Autodesk Inventor part; units mm, degrees
ref_plane "YZ Plane" through (0, 0, 0) normal (1, 0, 0) x (0, 1, 0)
ref_plane "XZ Plane" through (0, 0, 0) normal (0, 1, 0) x (-1, 0, 0)
ref_plane "XY Plane" through (0, 0, 0) normal (0, 0, 1) x (1, 0, 0)
ref_plane "작업 평면1" through (0, 0, -188.9899) normal (0, 0, 1) x (-0.9797373, 0.2002869, 0)
sketch "스케치1" plane through (0, 0, -188.9899) normal (0, 0, 1) x (-0.9797373, 0.2002869, 0)
  circle A0 centre (0, 0) radius 13.8
  circle A1 centre (0, 0) radius 7.2
  circle A2 centre (0, -11) radius 1.2813
  circle A3 centre (-7.7782, -7.7782) radius 1.2813
  circle A4 centre (-11, 0) radius 1.2813
  circle A5 centre (-7.7782, 7.7782) radius 1.2813
  circle A6 centre (0, 11) radius 1.2813
  circle A7 centre (7.7782, 7.7782) radius 1.2813
  circle A8 centre (11, 0) radius 1.2813
  circle A9 centre (7.7782, -7.7782) radius 1.2813
  line L0 (-17.5, -17.5) -> (17.5, -17.5)
  line L1 (17.5, -17.5) -> (17.5, 17.5)
  line L2 (17.5, 17.5) -> (-17.5, 17.5)
  line L3 (-17.5, 17.5) -> (-17.5, -17.5)
  line L4 (-17.5, -17.5) -> (17.5, 17.5) construction
  line L5 (17.5, -17.5) -> (-17.5, 17.5) construction
  circle A10 centre (0, 0) radius 7.3
  circle A11 centre (-11, 0) radius 1.3813
  circle A12 centre (-7.7782, 7.7782) radius 1.3813
  circle A13 centre (0, 11) radius 1.3813
  circle A14 centre (7.7782, 7.7782) radius 1.3813
  circle A15 centre (11, 0) radius 1.1813
  circle A16 centre (7.7782, -7.7782) radius 1.3813
  circle A17 centre (0, -11) radius 1.3813
  circle A18 centre (-7.7782, -7.7782) radius 1.3813
  line L6 (17.2724, -17.5) -> (17.2724, -18.1)
  line L7 (17.1076, 17.5) -> (17.1076, 22.85)
  line L8 (17.1076, 17.5) -> (22.4576, 17.5) construction
  line L9 (17.5, 22.85) -> (16.9, 22.85)
  line L10 (16.9, 22.85) -> (16.9, -18.1)
  line L11 (16.9, -18.1) -> (17.5, -18.1)
  line L12 (17.5, -18.1) -> (17.5, 22.85)
  line L13 (17.5, -18.1) -> (-17.5, -18.1)
  line L14 (-17.5, -18.1) -> (-17.5, 22.85)
  line L15 (-17.5, 22.85) -> (17.5, 22.85)
  line L16 (17.5, 22.85) -> (17.5, -18.1)
  line L17 (17.5, 17.5) -> (18.1, 17.5)
  line L18 (18.1, 17.5) -> (18.1, -17.5)
  line L19 (18.1, -17.5) -> (17.5, -17.5)
  line L20 (17.5, -17.5) -> (17.5, 17.5)
  line L21 (-17.5, 17.5) -> (-22.85, 17.5)
  line L22 (-22.85, 17.5) -> (-22.85, 15.9604)
  line L23 (-22.85, 15.9604) -> (-17.5, 15.9604)
  line L24 (-17.5, 15.9604) -> (-17.5, 17.5)
  line L25 (-22.85, 17.5) -> (-17.5, 17.5)
  line L26 (-17.5, 17.5) -> (-17.5, -17.5)
  line L27 (-17.5, -17.5) -> (-22.85, -17.5)
  line L28 (-22.85, -17.5) -> (-22.85, 17.5)
  point P0 (0, 0)
  point P1 (17.5, -17.5)
  point P2 (-17.5, -17.5)
  point P3 (16.9, -18.1)
  point P4 (16.9, 22.85)
  point P5 (-17.5, 17.5)
  point P6 (17.5, 17.5)
  point P7 (-22.85, 15.9604)
  point P8 (17.5, -17.5)
  dimension "d0" = 35
  dimension "d1" = 35
  dimension "d2" = 0.1
  dimension "d3" = 0.1
  dimension "d4" = 0.1
  dimension "d5" = 0.1
  dimension "d6" = 0.1
  dimension "d7" = 0.1
  dimension "d8" = 0.1
  dimension "d9" = 0.1
  dimension "d10" = 0.1
  dimension "d13" = 0.6
  dimension "d14" = 5.35
  dimension "d15" = 90
  dimension "d16" = 0.6
  dimension "d17" = 5.35
extrude "돌출1" add sketch "스케치1" along normal blind 6 contours A0 | L0 L10 L2 L1 | L1 L17 L18 L19 | L0 L3 L2 L10 | L27 L28 L23 L3 | L23 L22 L21 L3
sketch "스케치3" plane through (25.892, 12.5688, -182.9899) normal (0.9797373, -0.2002869, 0) x (0, 0, -1)
  circle A0 centre (2.59, -25.3) radius 1.55
  circle A1 centre (2.59, -9.7) radius 1.55
  line L0 (-34, -31.3) -> (6, -31.3)
  line L1 (6, -31.3) -> (6, -3.7)
  line L2 (6, -3.7) -> (-34, -3.7)
  arc A2 (-34, -3.7) -> (-34, -31.3) centre (-34, -17.5) ccw
  circle A3 centre (-41.7782, -25.2782) radius 1.65
  circle A4 centre (-45, -17.5) radius 1.65
  circle A5 centre (-41.7782, -9.7218) radius 1.65
  circle A6 centre (-34, -6.5) radius 1.65
  circle A7 centre (-26.2218, -9.7218) radius 1.65
  circle A8 centre (-23, -17.5) radius 1.65
  circle A9 centre (-26.2218, -25.2782) radius 1.65
  circle A10 centre (-34, -28.5) radius 1.65
  circle A11 centre (-34, -17.5) radius 5.1
  circle A12 centre (-34, -17.5) radius 3.9
  circle A13 centre (-34, -17.5) radius 4
  circle A14 centre (-28.3126, -11.8739) radius 1.2
  circle A15 centre (-39.6261, -11.8126) radius 1.2
  circle A16 centre (-39.6874, -23.1261) radius 1.2
  circle A17 centre (-28.3739, -23.1874) radius 1.2
  circle A18 centre (-34, -17.5) radius 4
  circle A19 centre (-34, -17.5) radius 10.9
  circle A20 centre (-34.0433, -25.4999) radius 1.2
  circle A21 centre (-41.9999, -17.4567) radius 1.2
  circle A22 centre (-33.9567, -9.5001) radius 1.2
  circle A23 centre (-26.0001, -17.5433) radius 1.2
  circle A24 centre (-34, -17.5) radius 3.5
  circle A25 centre (-34, -17.5) radius 5.2
  circle A26 centre (-26.0001, -17.5433) radius 1.3
  circle A27 centre (-28.3739, -23.1874) radius 1.3
  circle A28 centre (-34.0433, -25.4999) radius 1.3
  circle A29 centre (-39.6874, -23.1261) radius 1.3
  circle A30 centre (-41.9999, -17.4567) radius 1.3
  circle A31 centre (-39.6261, -11.8126) radius 1.3
  circle A32 centre (-33.9567, -9.5001) radius 1.3
  circle A33 centre (-28.3126, -11.8739) radius 1.3
  point P0 (-182.9899, -17.5)
  dimension "d22" = 0.1
  dimension "d23" = 0.1
  dimension "d24" = 0.1
  dimension "d25" = 0.1
  dimension "d26" = 0.1
  dimension "d27" = 0.1
  dimension "d28" = 0.1
  dimension "d29" = 0.1
  dimension "d30" = 0.1
  dimension "d31" = 0.1
extrude "돌출2" add sketch "스케치3" along normal blind 6 contours A0 | A1 | A2 L2 L1 L0 | A3 A19 | A3 A19 A4 A5 A6 A7 A8 A9 A10 | A19 A3 | A19 A4 | A4 A19 | A19 A10 | A10 A19 | A19 A5 | A5 A19 | A19 A9 | A9 A19 | A19 A6 | A6 A19 | A19 A8 | A8 A19 | A19 A7 | A7 A19 | A11 | A25
sketch "스케치4" plane through (-21.2383, -13.5202, -188.9899) normal (-0.9797373, 0.2002869, 0) x (0, 0, 1)
  circle A0 centre (3.41, 9.7) radius 1.55
  circle A1 centre (3.41, 25.3) radius 1.55
  line L0 (40, 3.7) -> (0, 3.7)
  arc A2 (40, 3.7) -> (40, 31.3) centre (40, 17.5) ccw
  line L1 (0, 31.3) -> (40, 31.3)
  line L2 (0, 3.7) -> (0, 31.3)
  circle A3 centre (47.7782, 9.7218) radius 1.65
  circle A4 centre (51, 17.5) radius 1.65
  circle A5 centre (47.7782, 25.2782) radius 1.65
  circle A6 centre (40, 28.5) radius 1.65
  circle A7 centre (32.2218, 25.2782) radius 1.65
  circle A8 centre (29, 17.5) radius 1.65
  circle A9 centre (32.2218, 9.7218) radius 1.65
  circle A10 centre (40, 6.5) radius 1.65
  circle A11 centre (40, 17.5) radius 5.1
  circle A12 centre (40, 17.5) radius 10.8
  circle A13 centre (40, 17.5) radius 6
  circle A14 centre (47.9984, 17.6612) radius 1.05
  circle A15 centre (45.7697, 11.9583) radius 1.05
  circle A16 centre (40.1612, 9.5016) radius 1.05
  circle A17 centre (34.4583, 11.7303) radius 1.05
  circle A18 centre (32.0016, 17.3388) radius 1.05
  circle A19 centre (34.2303, 23.0417) radius 1.05
  circle A20 centre (39.8388, 25.4984) radius 1.05
  circle A21 centre (45.5417, 23.2697) radius 1.05
  circle A22 centre (39.8388, 25.4984) radius 1.15
  circle A23 centre (34.2303, 23.0417) radius 1.15
  circle A24 centre (32.0016, 17.3388) radius 1.15
  circle A25 centre (34.4583, 11.7303) radius 1.15
  circle A26 centre (40.1612, 9.5016) radius 1.15
  circle A27 centre (45.7697, 11.9583) radius 1.15
  circle A28 centre (47.9984, 17.6612) radius 1.15
  circle A29 centre (45.5417, 23.2697) radius 1.15
  point P0 (188.9899, 17.5)
  dimension "d32" = 0.1
  dimension "d33" = 0.1
  dimension "d34" = 0.1
  dimension "d35" = 0.1
  dimension "d36" = 0.1
  dimension "d37" = 0.1
  dimension "d38" = 0.1
  dimension "d39" = 0.1
extrude "돌출3" add sketch "스케치4" along normal blind 6 contours A0 | A1 | L0 L2 L1 A2 | A3 A12 | A12 A3 | A3 A12 A10 A9 A8 A7 A6 A5 A4 | A12 A4 | A4 A12 | A12 A10 | A10 A12 | A12 A5 | A5 A12 | A12 A9 | A9 A12 | A12 A6 | A6 A12 | A12 A8 | A8 A12 | A12 A7 | A7 A12 | A13
sketch "스케치5" plane through (0, 0, -182.9899) normal (0, 0, 1) x (0.9797373, -0.2002869, 0)
  line L0 (22.85, 13.8) -> (22.85, -13.8)
  line L1 (22.85, -13.8) -> (28.85, -13.8)
  line L2 (28.85, 13.8) -> (28.85, -13.8)
  line L3 (22.85, 13.8) -> (28.85, 13.8)
  line L4 (-18.1, -13.8) -> (-18.1, 13.8)
  line L5 (-18.1, 13.8) -> (-24.1, 13.8)
  line L6 (-24.1, -13.8) -> (-24.1, 13.8)
  line L7 (-18.1, -13.8) -> (-24.1, -13.8)
  line L8 (22.85, -17.5) -> (22.85, -13.8)
  line L9 (-18.1, -13.8) -> (-18.1, -17.5)
  line L10 (22.85, -13.8) -> (-18.1, -13.8)
  line L11 (-18.1, -13.8) -> (-18.1, -17.5)
  line L12 (-18.1, -17.5) -> (22.85, -17.5)
  line L13 (22.85, -17.5) -> (22.85, -13.8)
  line L14 (-18.1, -17.5) -> (22.85, -17.5)
  line L15 (22.85, -17.5) -> (22.85, -13.8)
  line L16 (22.85, -13.8) -> (22.85, 13.8)
  line L17 (22.85, 13.8) -> (22.85, 17.5)
  line L18 (22.85, 17.5) -> (-18.1, 17.5)
  line L19 (-18.1, 17.5) -> (-18.1, 13.8)
  line L20 (-18.1, 13.8) -> (-18.1, -13.8)
  line L21 (-18.1, -13.8) -> (-18.1, -17.5)
  circle A0 centre (-11, 0) radius 1.2813
  circle A1 centre (0, 0) radius 7.3
  circle A2 centre (11, 0) radius 1.3813
  circle A3 centre (7.7782, -7.7782) radius 1.3813
  circle A4 centre (0, -11) radius 1.3813
  circle A5 centre (-7.7782, -7.7782) radius 1.3813
  circle A6 centre (-7.7782, 7.7782) radius 1.3813
  circle A7 centre (0, 11) radius 1.3813
  circle A8 centre (7.7782, 7.7782) radius 1.3813
  line L22 (22.85, 13.8) -> (-18.3673, 13.8)
  line L23 (-18.3673, 13.8) -> (-18.3673, 17.5)
  line L24 (-18.3673, 17.5) -> (22.85, 17.5)
  line L25 (22.85, 17.5) -> (22.85, 13.8)
  point P0 (0, 0)
  point P1 (-18.1, 13.8)
  point P2 (-18.1, -13.8)
  point P3 (22.85, -17.5)
extrude "돌출4" cut sketch "스케치5" against normal blind 10 contours L22 L19 L18 L17 | L8 L12 L9 L10
properties part number "37" material "LCP 플라스틱"
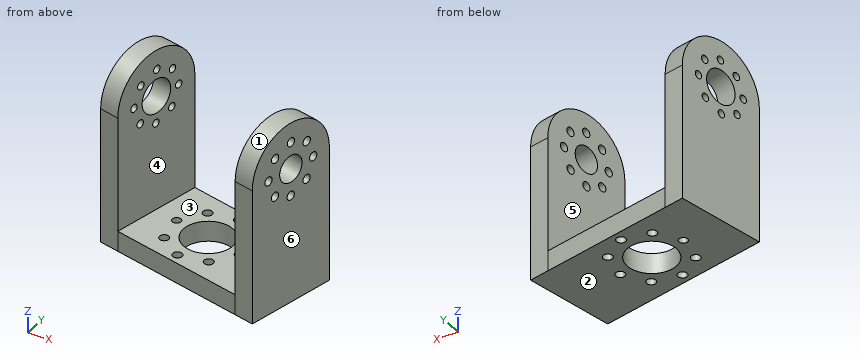
Source: CAD feature listing. Evaluate the final solid. Frame: model axes, mm. Face numbers are marked on the shaded views. A direction names the side the tool comes from. Give positions to 0.01 mm unless a question says otherwise; leave off trailing zeros. Loops run counter-clockwise (first coordinate to the right, second up) from the corner with the lowest first, then second, coordinate; pieces in that order, holes last. Notation, with made-up numbers: (-38.75, -8) -> (-11.75, -8) arc R23 ccw to (-11.75, 6) -> close; hole circle Ø9 at (-0.75, 55). An arc over 180 degrees is marked (long way). Use a Markdown table: item, result. Add a question column.
(1) First-contact query: pin 1 Ø3 at (x, y) = (0, -10) entering from +Z; pin 2 Ø8 at (x, z) = (-6.5, -177.5) entering from -Y; pin 3 Ø1.5 at (x, z) = (-20, -176.5) entering from -Y; pin 4 Ø8 at (y, z) = (-6, -149.5) entering from +X. Flat tips, straight axial feed; report the tip coordinate or a pass-through.
(2) Section query A-A (z = -172). Output: boundary loops of the cut face in (x, y), then the cut area to 3 significant figures.
(3) Section query D-D (z = -146.5). Output: boundary loops of the cut face in (x, y).
(4) Pull-direction query (X, two-part tool) for the marked faces 1, 2 and 3; classes: +X half, -X half, draft (parallel to the pull), parting line (faces both ways), or undercut.
(5) Access query for the marked faces 4, 5 and 6. Directions: +Z, -Z, +X, -X, +Y, -Y. A direction counts if a zero-diameter tool reaches every point of the face in a straight line with its end or side. Return the directions, or none.
(6) Section query C-C (x = -8.5). Output: boundary loops of the cut face in (y, z).
(7) Ray query, line 1 (Z direction, x = 25, y = -11); line 2 (Z direction, x = 8, y = 10.5); line 3 (X direction, y = 0, z = -186.65). Return the intervals inside material, ascending.
(8) Section query B-B (x = 6). Output: boundary loops of the cut face in (y, z), then the cut area to 3 significant figures.
Checked values:
| question | item | result |
|---|---|---|
| 1 | pin 1 | z = -182.99 |
| 1 | pin 2 | through |
| 1 | pin 3 | y = -9.9 |
| 1 | pin 4 | x = 29.02 |
| 2 | outline | (-26.38, -8.69) -> (-20.5, -9.9) -> (-14.97, 17.15) -> (-20.85, 18.35) -> close; (19.62, -18.1) -> (25.5, -19.3) -> (31.03, 7.74) -> (25.15, 8.94) -> close |
| 2 | area | 331 mm^2 |
| 3 | outline | (-26.33, -8.47) -> (-20.45, -9.67) -> (-18.62, -0.74) -> (-24.5, 0.47) -> close; (-22.72, 9.19) -> (-16.84, 7.99) -> (-15.01, 16.92) -> (-20.89, 18.13) -> close; (19.67, -17.88) -> (25.55, -19.08) -> (27.64, -8.85) -> (21.76, -7.64) -> close; (23.01, -1.51) -> (28.89, -2.71) -> (30.98, 7.52) -> (25.11, 8.72) -> close |
| 4 | face 1 | parting line |
| 4 | face 2 | draft |
| 4 | face 3 | undercut |
| 5 | face 4 | +Z, -Y |
| 5 | face 5 | +Z, +Y |
| 5 | face 6 | +Z, -Z, +X, -Y |
| 6 | outline | (-12.35, -188.99) -> (-7.27, -188.99) -> (-7.27, -182.99) -> (-12.35, -182.99) -> close; (-4.86, -188.99) -> (15.82, -188.99) -> (15.82, -182.99) -> (-4.86, -182.99) -> close |
| 7 | line 1 | -188.99 to -155.91, -153.32 to -144.59, -142.01 to -136.45 |
| 7 | line 2 | -188.99 to -182.99 |
| 7 | line 3 | -24.6 to -7.3, 7.3 to 29.45 |
| 8 | outline | (-15.31, -188.99) -> (-10.56, -188.99) -> (-10.56, -182.99) -> (-15.31, -182.99) -> close; (-7.8, -188.99) -> (-4.16, -188.99) -> (-4.16, -182.99) -> (-7.8, -182.99) -> close; (4.16, -188.99) -> (12.86, -188.99) -> (12.86, -182.99) -> (4.16, -182.99) -> close |
| 8 | area | 103 mm^2 |
